Here's the drawing with two shaded views (mm, measured from the low corner). I have some questions. A direction names the side the tool comes from. Coordinates: 2 decimals unless noted, no trailing zeros. Loops run counter-clockwise (first coordinate to the right, second up) from the corner with the lowest first, then second, coordinate; pieces in that order, holes last. Notation, with made-up numbers: (9.5, 52) - (28.5, 52) arc R20 cw to (28.5, 80) - close; hole circle Ø10 at (-28, 65). An arc over 180 degrees is marked (long way). Use a Markdown table: item, result.
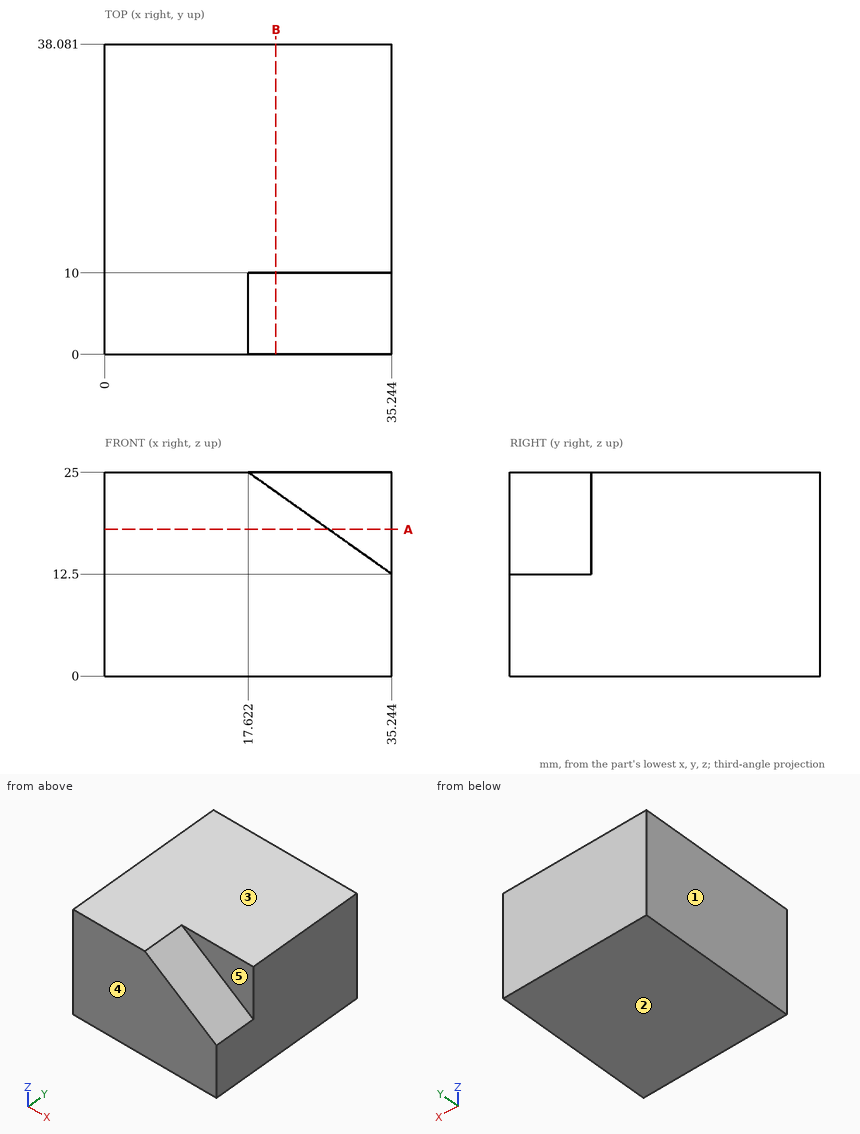
Q1. I want a section at A-A, the plane z = 18. Write out the boundary of the cut face in (x, y).
Check values:
| item | result |
|---|---|
| outline | (0, 0) - (27.49, 0) - (27.49, 10) - (35.24, 10) - (35.24, 38.08) - (0, 38.08) - close |
Q2. If we mould it in two halves opening along Z, with no side actions, what happens to the marked faces 1, 2 and 3? For each: pulls with the +Z half, pulls with the -Z half, needs draft (parallel to the pull), parting line crosses it, or undercut.
Check values:
| item | result |
|---|---|
| face 1 | needs draft |
| face 2 | pulls with the -Z half |
| face 3 | pulls with the +Z half |
Q3. Please list where these lines run through material, in increasing order: L1, parallel to Z at x = 22, y = 2.5 (1 decimal); L2, parallel to Z at x = 30, y = 7.5; L3, parallel to X at y = 2.5, z = 23.25. Write a range as from..to.
Check values:
| item | result |
|---|---|
| L1 | 0..21.9 |
| L2 | 0..16.22 |
| L3 | 0..20.09 |
Q4. I want a section at B-B, the plane x = 21. Write out the boundary of the cut face in (y, z), then the cut area to 3 significant figures.
Check values:
| item | result |
|---|---|
| outline | (0, 0) - (38.08, 0) - (38.08, 25) - (10, 25) - (10, 22.6) - (0, 22.6) - close |
| area | 928 mm^2 |
Q5. Which directions (+Z, -Z, +X, -X, +Y, -Y) give clear straight access to the entire face, cutting with the end or side of a thin tool? Please do the marked faces 4 and 5.
Check values:
| item | result |
|---|---|
| face 4 | +Z, -Z, +X, -X, -Y |
| face 5 | +Z, +X, -Y |
